from build123d import *

# Parameters (mm, degrees)
F0_R     = 1.55
F0_R_2   = 2
F0_R_3   = 10.5
F0_R_4   = 1.5
F0_R_5   = 5.1
F1_DEPTH = 10


with BuildPart() as f1:
    # F0 (on Top) → F1 (new body)
    with BuildSketch(Plane.XY):
        with BuildLine():
            ThreePointArc((-81.7, 150.05), (-85.235534, 148.585534), (-86.7, 145.05))
            Line((-86.7, 145.05), (-86.7, 72.95))
            ThreePointArc((-86.7, 72.95), (-88.164466, 69.414466), (-91.7, 67.95))
            Line((-91.7, 67.95), (-104.5, 67.95))
            ThreePointArc((-104.5, 67.95), (-108.035534, 66.485534), (-109.5, 62.95))
            Line((-109.5, 62.95), (-109.5, -146.05))
            ThreePointArc((-109.5, -146.05), (-108.035534, -149.585534), (-104.5, -151.05))
            Line((-104.5, -151.05), (104.5, -151.05))
            ThreePointArc((104.5, -151.05), (108.035534, -149.585534), (109.5, -146.05))
            Line((109.5, -146.05), (109.5, 62.95))
            ThreePointArc((109.5, 62.95), (108.035534, 66.485534), (104.5, 67.95))
            Line((104.5, 67.95), (91.7, 67.95))
            ThreePointArc((91.7, 67.95), (88.164466, 69.414466), (86.7, 72.95))
            Line((86.7, 72.95), (86.7, 145.05))
            ThreePointArc((86.7, 145.05), (85.235534, 148.585534), (81.7, 150.05))
            Line((81.7, 150.05), (-81.7, 150.05))
        make_face()
        with Locations((-104.5, -146.05)):
            Circle(F0_R, mode=Mode.SUBTRACT)
        Polygon((-96.5, -125.559945), (-96.5, -49.554576), (-20.49463, -49.554576), align=None, mode=Mode.SUBTRACT)
        Polygon((-84.009945, -138.05), (-8.004576, -62.04463), (-8.004576, -138.05), align=None, mode=Mode.SUBTRACT)
        Polygon((8.004576, -62.04463), (84.009945, -138.05), (8.004576, -138.05), align=None, mode=Mode.SUBTRACT)
        with Locations((104.5, -146.05)):
            Circle(F0_R, mode=Mode.SUBTRACT)
        Polygon((96.5, -49.554576), (96.5, -125.559945), (20.49463, -49.554576), align=None, mode=Mode.SUBTRACT)
        Polygon((-96.5, -33.545424), (-96.5, 42.459945), (-20.49463, -33.545424), align=None, mode=Mode.SUBTRACT)
        with Locations((-104.5, 62.95)):
            Circle(F0_R, mode=Mode.SUBTRACT)
        Polygon((-8.004576, -21.05537), (-84.009945, 54.95), (-8.004576, 54.95), align=None, mode=Mode.SUBTRACT)
        with Locations((-69.313708, 118.636292)):
            Circle(F0_R_2, mode=Mode.SUBTRACT)
        with Locations((-58, 129.95)):
            Circle(F0_R_3, mode=Mode.SUBTRACT)
        with Locations((-69.313708, 141.263708)):
            Circle(F0_R_2, mode=Mode.SUBTRACT)
        with Locations((-46.686292, 118.636292)):
            Circle(F0_R_2, mode=Mode.SUBTRACT)
        with Locations((-46.686292, 141.263708)):
            Circle(F0_R_2, mode=Mode.SUBTRACT)
        with Locations((-8, 129.95)):
            Circle(F0_R_4, mode=Mode.SUBTRACT)
        Polygon((84.009945, 54.95), (8.004576, -21.05537), (8.004576, 54.95), align=None, mode=Mode.SUBTRACT)
        with Locations((0, 62.95)):
            Circle(F0_R, mode=Mode.SUBTRACT)
        Polygon((96.5, -33.545424), (20.49463, -33.545424), (96.5, 42.459945), align=None, mode=Mode.SUBTRACT)
        with Locations((104.5, 62.95)):
            Circle(F0_R, mode=Mode.SUBTRACT)
        with Locations((0, 121.95)):
            Circle(F0_R_4, mode=Mode.SUBTRACT)
        with Locations((0, 129.95)):
            Circle(F0_R_5, mode=Mode.SUBTRACT)
        with Locations((8, 129.95)):
            Circle(F0_R_4, mode=Mode.SUBTRACT)
        with Locations((0, 137.95)):
            Circle(F0_R_4, mode=Mode.SUBTRACT)
        with Locations((46.686292, 118.636292)):
            Circle(F0_R_2, mode=Mode.SUBTRACT)
        with Locations((46.686292, 141.263708)):
            Circle(F0_R_2, mode=Mode.SUBTRACT)
        with Locations((58, 129.95)):
            Circle(F0_R_3, mode=Mode.SUBTRACT)
        with Locations((69.313708, 118.636292)):
            Circle(F0_R_2, mode=Mode.SUBTRACT)
        with Locations((69.313708, 141.263708)):
            Circle(F0_R_2, mode=Mode.SUBTRACT)
    extrude(amount=F1_DEPTH)


solid = f1.part
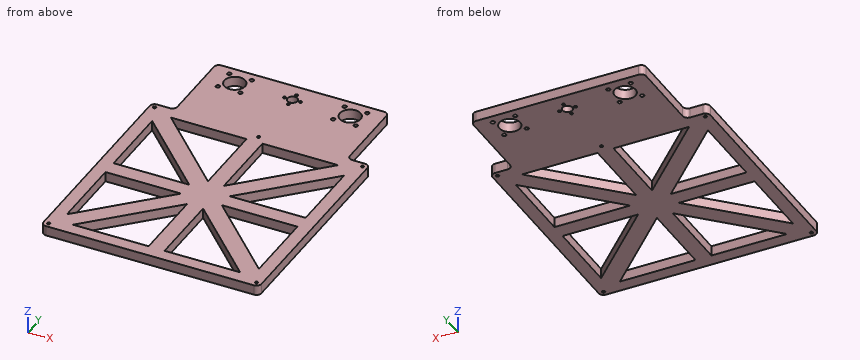
For this review, take the finished solid that the model builds, in its own axes (mm). Coordinates: 2 decimals unless noted, no trailing zeros. Loops run counter-clockwise (first coordinate to the right, second up) from the corner with the lowest first, then second, coordinate; pieces in that order, holes last. Notation, with made-up numbers: (25, 18) - (46, 18) arc R28 cw to (46, 50) - close; hole circle Ø8 at (-3.5, 84.5). An arc over 180 degrees is marked (long way). Return JSON: item names as keys, results as strings.
Item 1: Insertion check: pin 1 (5 mm diameter, centred on y = 99, z = 2, fed in from -X); pin 2 (5 mm diameter, centred on x = -46.69, y = 141.26, fed in from -Z). Each pin has a flat end and moves straight along its axis. Give the tip position at first contact, or say it passes through.
Determined:
{"pin 1": "stops at x = -86.7", "pin 2": "stops at z = 0"}
Item 2: For line 1 (Y direction, x = 0, z = 6.5); line 2 (X direction, y = 11, z = 5.75); line 3 (Y direction, x = 104.5, z = 8), list the stretches that pass through material, from the lowest coordinate up.
Determined:
{"line 1": "y = -151.05 to 61.4, 64.5 to 120.45, 123.45 to 124.85, 135.05 to 136.45, 139.45 to 150.05", "line 2": "x = -109.5 to -96.5, -65.04 to -40.06, -8 to 8, 40.06 to 65.04, 96.5 to 109.5", "line 3": "y = -151.05 to -147.6, -144.5 to 61.4, 64.5 to 67.95"}
Item 3: Take a section at C-C (y = 29). Give the boundary of the cut face in (x, z), then the cut area to 3 significant figures.
Determined:
{"outline": "(-109.5, 0) - (-96.5, 0) - (-96.5, 10) - (-109.5, 10) - close; (-83.04, 0) - (-58.06, 0) - (-58.06, 10) - (-83.04, 10) - close; (-8, 0) - (8, 0) - (8, 10) - (-8, 10) - close; (58.06, 0) - (83.04, 0) - (83.04, 10) - (58.06, 10) - close; (96.5, 0) - (109.5, 0) - (109.5, 10) - (96.5, 10) - close", "area": "920 mm2"}
Item 4: Take a section at D-D (z = 8.5). State how many separate pieces and enclosed holes the cut face has, then the cut area to 3 significant figures.
Determined:
{"separate pieces": "1", "enclosed holes": "28", "area": "38,100 mm2"}
Item 5: Take a section at A-A (x = -58). Give the boundary of the cut face in (y, z).
Determined:
{"outline": "(-151.05, 0) - (-138.05, 0) - (-138.05, 10) - (-151.05, 10) - close; (-112.04, 0) - (-87.06, 0) - (-87.06, 10) - (-112.04, 10) - close; (-49.55, 0) - (-33.55, 0) - (-33.55, 10) - (-49.55, 10) - close; (3.96, 0) - (28.94, 0) - (28.94, 10) - (3.96, 10) - close; (54.95, 0) - (119.45, 0) - (119.45, 10) - (54.95, 10) - close; (140.45, 0) - (150.05, 0) - (150.05, 10) - (140.45, 10) - close"}
Item 6: Take a section at B-B (x = 77). Give the boundary of the cut face in (y, z).
Determined:
{"outline": "(-151.05, 0) - (-138.05, 0) - (-138.05, 10) - (-151.05, 10) - close; (-131.04, 0) - (-106.06, 0) - (-106.06, 10) - (-131.04, 10) - close; (-49.55, 0) - (-33.55, 0) - (-33.55, 10) - (-49.55, 10) - close; (22.96, 0) - (47.94, 0) - (47.94, 10) - (22.96, 10) - close; (54.95, 0) - (150.05, 0) - (150.05, 10) - (54.95, 10) - close"}
